Design review of the part built by this model. Coordinates are the model's own, in mm. Round coordinates to 2 decimals unless told otherwise and drop trailing zeros. Write each loop counter-clockwise with the first axis right and the second up, starting at its lowest first coordinate (ties: lowest second). Pieces come first, ordered by that corner, then holes. Notation, with made-up numbers: (-12.5, 12) - (12.5, 12) arc R18 cw to (12.5, 22) - close; hole circle Ø4 at (-39.5, 13.25). An arc over 180 degrees is marked (long way). Use one line per item in the form item = value.
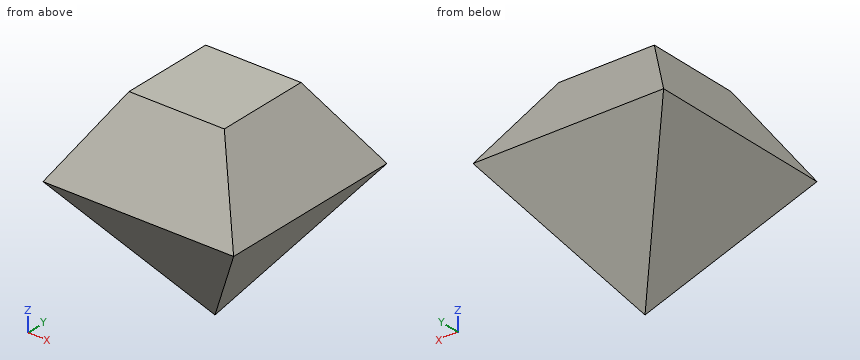
```python
from build123d import *

# Parameters (mm, degrees)
F0_W     = 91.44
F0_H     = 116.84
F1_DEPTH = 91.44
F4_DEPTH = 127
F5_DEPTH = 152.4


with BuildPart() as f1:
    # F0 (on Front) → F1 (new body)
    with BuildSketch(Plane.XZ):
        with Locations((0, -2.535963)):
            Rectangle(F0_W, F0_H)
    extrude(amount=F1_DEPTH)

    # F2 (on face) → F4 (cut)
    with BuildSketch(Plane.XZ.offset(91.44)):
        Polygon((-45.72, 55.884037), (-45.72, 0), (-22.86, 36.632401), (22.86, 36.632401), (45.72, 0), (45.72, 55.884037), align=None)
        Polygon((45.72, 0), (0, -60.955963), (45.72, -60.955963), align=None)
        Polygon((-45.72, -60.955963), (0, -60.955963), (-45.72, 0), align=None)
    extrude(amount=-F4_DEPTH, mode=Mode.SUBTRACT)

    # F3 (on face) → F5 (cut)
    with BuildSketch(Plane.YZ.offset(45.72)):
        Polygon((-91.44, 55.884037), (-91.44, 0), (-68.58, 36.632401), (-22.86, 36.632401), (0, 0), (0, 55.884037), align=None)
        Polygon((0, 0), (-45.72, -60.955963), (0, -60.955963), align=None)
        Polygon((-91.44, -60.955963), (-45.72, -60.955963), (-91.44, 0), align=None)
    extrude(amount=-F5_DEPTH, mode=Mode.SUBTRACT)


solid = f1.part
```
Q1. We need section A-A on y = -43. Write out the cut boundary in (x, z).
Calculated:
outline = (-45.72, 0) - (-2.72, -57.33) - (2.72, -57.33) - (45.72, 0) - (22.86, 36.63) - (-22.86, 36.63) - close
Q2. We need section D-D on z = -39.5. Write out the cut boundary in (x, y), then the cut area to 3 significant figures.
Calculated:
outline = (-16.09, -61.81) - (16.09, -61.81) - (16.09, -29.63) - (-16.09, -29.63) - close
area = 1,040 mm2
Q3. For P1, Ø2, axis at x = 0, z = -12.5, coming from the +Y side; P2, Ø3, axis at x = 4.5, y = -37, coming from the -Z side; P3, Ø10, axis at y = -31.5, z = 11.5, coming from the -X side, all flat-tipped, find the tip position at first contact; note any pin that passes through.
Calculated:
P1 = -8.63
P2 = -51.33
P3 = -41.66
Q4. To check wall thickness, follow line 1 along X through (y, z) = (-49, -30.5); line 2 along X through (y, z) = (-72, 26); line 3 along Z through (x, y) = (-3.5, -78). State the ranges of each line that lie inside material, in increasing order. Write a range as from..to.
Calculated:
line_1 = -22.84..22.84
line_2 = -29.5..29.5
line_3 = -17.92..21.54
Q5. We need section B-B on x = 31.5. Write out the cut boundary in (y, z).
Calculated:
outline = (-91.44, 0) - (-77.22, -18.96) - (-14.22, -18.96) - (0, 0) - (-14.22, 22.79) - (-77.22, 22.79) - close
Q6. We need section C-C on z = 3. Write out the cut boundary in (x, y).
Calculated:
outline = (-43.85, -89.57) - (43.85, -89.57) - (43.85, -1.87) - (-43.85, -1.87) - close
